```python
from build123d import *

# Parameters (mm, degrees)
SKETCH1_W           = 109.5
SKETCH1_H           = 26
BOSS_EXTRUDE2_DEPTH = 15
BOSS_EXTRUDE5_DEPTH = 9.5
BOSS_EXTRUDE6_DEPTH = 13
SKETCH2_W           = 6.5
SKETCH2_H           = 11.5
CUT_EXTRUDE1_DEPTH  = 171.414201286
FILLET1_R           = 2.5


with BuildPart() as part:
    # Sketch1 → Boss-Extrude2 (new, symmetric)
    with BuildSketch(Plane(origin=(0, 0, 0), x_dir=(1, 0, 0), z_dir=(0, 1, 0))):
        with Locations((54.75, 0)):
            Rectangle(SKETCH1_W, SKETCH1_H)
    extrude(amount=BOSS_EXTRUDE2_DEPTH, both=True)

    # Sketch1<6> → Boss-Extrude5 (add, symmetric)
    # profile 1 of 2: a face of its own
    with BuildSketch(Plane(origin=(0, 0, 0), x_dir=(1, 0, 0), z_dir=(0, 1, 0))):
        Polygon((0, -30.5), (0, -48), (105, -48), (105, -31), (133, -31), (115, -13), (0, -13), align=None)
        with BuildLine():
            ThreePointArc((30.5, -35.5), (26.964466094, -34.035533906), (25.5, -30.5))
            ThreePointArc((25.5, -30.5), (26.964466094, -26.964466094), (30.5, -25.5))
            Line((30.5, -25.5), (81.5, -25.5))
            ThreePointArc((81.5, -25.5), (86.5, -30.5), (81.5, -35.5))
            Line((81.5, -35.5), (30.5, -35.5))
        make_face(mode=Mode.SUBTRACT)
    # profile 2 of 2: a face of its own
    with BuildSketch(Plane(origin=(0, 0, 0), x_dir=(1, 0, 0), z_dir=(0, 1, 0))):
        Polygon((0, 30.5), (0, 13), (115, 13), (133, 31), (105, 31), (105, 48), (0, 48), align=None)
        with BuildLine():
            ThreePointArc((30.5, 25.5), (26.964466094, 26.964466094), (25.5, 30.5))
            ThreePointArc((25.5, 30.5), (26.964466094, 34.035533906), (30.5, 35.5))
            Line((30.5, 35.5), (81.5, 35.5))
            ThreePointArc((81.5, 35.5), (86.5, 30.5), (81.5, 25.5))
            Line((81.5, 25.5), (30.5, 25.5))
        make_face(mode=Mode.SUBTRACT)
    extrude(amount=BOSS_EXTRUDE5_DEPTH, both=True)

    # Sketch1<7> → Boss-Extrude6 (add, symmetric)
    with BuildSketch(Plane(origin=(0, 0, 0), x_dir=(1, 0, 0), z_dir=(0, 1, 0))):
        Polygon((105, -31), (105, -48), (140, -48), (140, -38), (133, -31), align=None)
        Polygon((140, 48), (105, 48), (105, 31), (133, 31), (140, 38), align=None)
    extrude(amount=BOSS_EXTRUDE6_DEPTH, both=True)

    # Sketch2 → Cut-Extrude1 (cut, through all)
    with BuildSketch(Plane(origin=(0, 0, -48), x_dir=(-1, 0, 0), z_dir=(0, 0, -1))):
        with Locations((-3.25, 9.25)):
            Rectangle(SKETCH2_W, SKETCH2_H)
    extrude(amount=-CUT_EXTRUDE1_DEPTH, mode=Mode.SUBTRACT)

    # Fillet1
    fillet1_edges = [part.edges().sort_by_distance(p)[0] for p in [
        (25.5, 9.5, -30.5),
        (56, -9.5, -35.5),
        (86.5, 9.5, -30.5),
        (56, 9.5, -25.5),
        (56, 9.5, -35.5),
        (25.5, -9.5, -30.5),
        (56, -9.5, -25.5),
        (86.5, -9.5, -30.5),
        (25.5, -9.5, 30.5),
        (56, -9.5, 25.5),
        (86.5, -9.5, 30.5),
        (56, 9.5, 35.5),
        (25.5, 9.5, 30.5),
        (56, 9.5, 25.5),
        (86.5, 9.5, 30.5),
        (56, -9.5, 35.5),
    ]]
    fillet(fillet1_edges, radius=FILLET1_R)


solid = part.part
```
Design review of the part built by this model. Coordinates are the model's own, in mm. A direction names the side the tool comes from. Coordinates: 2 decimals unless noted, no trailing zeros. Order: outer loops, then holes, each group sorted by start corner. A loop starts at its lowest first (then second) coordinate and runs counter-clockwise, first axis right, second up. Notation, with made-up numbers: (84, 63.25) -> (127, 63.25) arc R10 ccw to (127, 77.25) -> close; hole circle Ø1 at (-37, 55). An arc over 180 degrees is marked (long way). One line per item, written item: value. Start each with the question number.
Q1. Take a section at B-B, the plane x = 117. State the section outline as (y, z) points.
Q2. Take a section at C-C, the plane y = 11. State the section outline as (x, z) points, then the cut area to 3 significant figures.
Q3. Take a section at D-D, the plane z = -4. State the section outline as (x, y) points, then the cut area to 3 significant figures.
Q4. Mouldability with a two-part tool opening along X and no side actions: class faces 4 (the flat face through (51, -9.5, 22)), 5 (the flat face through (140, 0, 43)), 6 (the flat face through (56, 0, -35.5)) as pulls with the +X half, pulls with the -X half, needs draft (parallel to the pull), parting line crosses it, or undercut.
Q5. For probe 1 along Z at (x, y) = (34, -6.75); probe 2 along Z at (x, y) = (30, 9.25); probe 3 along Z at (x, y) = (121, -10), list the stretches that pass through material, from the lowest coordinate up.
Q6. Tool access review of faces 1 (the cylindrical face through (25.5, -0.1, -30.4)), 2 (the flat face through (105, 11, -40)), 3 (the flat face through (105, -11, 39)): name each direction out of +Z, -Z, +X, -X, +Y, -Y from which nothing blocks a thin tool from reaching the whole face with its end or side.
Q7. Insertion check: pin 1 Ø1.6 at (x, y) = (72, 13) entering from -Z; pin 2 Ø10 at (y, z) = (-8, 14.5) entering from +X; pin 3 Ø6 at (y, z) = (5.5, -19) entering from +X. Each pin has a flat end and moves straight along its axis. Give the tip position at first contact, or say it passes through.
Q8. Take a section at A-A, the plane x = 34.5. State the section outline as (y, z) points, then the cut area to 3 significant figures.
Values follow:
1. outline: (-13, -48) -> (13, -48) -> (13, -31) -> (9.5, -31) -> (9.5, -15) -> (-9.5, -15) -> (-9.5, -31) -> (-13, -31) -> close; (-13, 31) -> (-9.5, 31) -> (-9.5, 15) -> (9.5, 15) -> (9.5, 31) -> (13, 31) -> (13, 48) -> (-13, 48) -> close
2. outline: (6.5, -13) -> (109.5, -13) -> (109.5, 13) -> (6.5, 13) -> close; (105, -48) -> (140, -48) -> (140, -38) -> (133, -31) -> (105, -31) -> close; (105, 31) -> (133, 31) -> (140, 38) -> (140, 48) -> (105, 48) -> close
2. area: 3,820 mm2
3. outline: (0, -15) -> (109.5, -15) -> (109.5, 15) -> (6.5, 15) -> (6.5, 3.5) -> (0, 3.5) -> close
3. area: 3,210 mm2
4. face 4: needs draft
4. face 5: pulls with the +X half
4. face 6: undercut
5. probe 1: z = -48 to -35.5, -25.5 to 25.5, 35.5 to 48
5. probe 2: z = -48 to -36.89, -24.11 to 24.11, 36.89 to 48
5. probe 3: z = -48 to -31, 31 to 48
6. face 1: +Y, -Y
6. face 2: -Z, -X, +Y
6. face 3: +Z, -X, -Y
7. pin 1: stops at z = -13
7. pin 2: stops at x = 121.5
7. pin 3: stops at x = 124
8. outline: (-15, -13) -> (-9.5, -13) -> (-9.5, -23) arc R2.5 ccw to (-7, -25.5) -> (7, -25.5) arc R2.5 ccw to (9.5, -23) -> (9.5, -13) -> (15, -13) -> (15, 13) -> (9.5, 13) -> (9.5, 23) arc R2.5 ccw to (7, 25.5) -> (-7, 25.5) arc R2.5 ccw to (-9.5, 23) -> (-9.5, 13) -> (-15, 13) -> close; (-9.5, -48) -> (9.5, -48) -> (9.5, -38) arc R2.5 ccw to (7, -35.5) -> (-7, -35.5) arc R2.5 ccw to (-9.5, -38) -> close; (-9.5, 38) arc R2.5 ccw to (-7, 35.5) -> (7, 35.5) arc R2.5 ccw to (9.5, 38) -> (9.5, 48) -> (-9.5, 48) -> close
8. area: 1,720 mm2
